from build123d import *

# Parameters (mm, degrees)
F0_W     = 100
F0_H     = 60
F1_DEPTH = 50
F2_W     = 15
F2_H     = 32
F3_DEPTH = 100.001
F4_W     = 70
F4_H     = 15
F5_DEPTH = 60.001
F6_SIZE2 = 15
F6_SIZE  = 20
F7_SIZE2 = 40
F7_SIZE  = 44


with BuildPart() as f1:
    # F0 (on Front) → F1 (new body)
    with BuildSketch(Plane.XZ):
        with Locations((50, 30)):
            Rectangle(F0_W, F0_H)
    extrude(amount=F1_DEPTH)

    # F2 (on face) → F3 (cut, through all)
    with BuildSketch(Plane.YZ.offset(100)):
        with Locations((-42.5, 16)):
            Rectangle(F2_W, F2_H)
    extrude(amount=-F3_DEPTH, mode=Mode.SUBTRACT)

    # F4 (on face) → F5 (cut, through all)
    with BuildSketch(Plane.XY.offset(60)):
        with Locations((65, -7.5)):
            Rectangle(F4_W, F4_H)
    extrude(amount=-F5_DEPTH, mode=Mode.SUBTRACT)

    # F6
    f6_edges = [f1.edges().sort_by_distance(p)[0] for p in [
        (0, -25, 60),
    ]]
    chamfer(f6_edges, length=F6_SIZE, length2=F6_SIZE2)

    # F7
    f7_edges = [f1.edges().sort_by_distance(p)[0] for p in [
        (100, -32.5, 60),
    ]]
    chamfer(f7_edges, length=F7_SIZE, length2=F7_SIZE2)


solid = f1.part
Input: part model. Units: mm. Frame: model coordinates. A direction names the side the tool comes from. Give positions to 0.01 mm unless a question says otherwise; leave off trailing zeros. Write each loop counter-clockwise with the first axis right and the second up, starting at its lowest first coordinate (ties: lowest second). Pieces come first, ordered by that corner, then holes. Notation, with made-up numbers: M 18.5,65.5 L 48.5,65.5 A15 ccw 48.5,80.5 Z; hole C 9,63.25 d4. An arc over 180 degrees is marked long. Write item = value, one per line. Start each with the question number.
1) Cut plane C-C on x = 19. Return the cut outline in (y, z), then the cut area to 3 significant figures.
2) Cut plane D-D on y = -3. Return the cut outline in (x, z), then the cut area to 3 significant figures.
3) Reachability of faces 1 (the flat face through (73.419, -32.255, 44.164)), 2 (the flat face through (51, -35, 16)), 3 (the flat face through (30, -8, 30)) from +Z, -Z, +X, -X, +Y, -Y: full face, straight path, thin tool, end or side. Return the list, or none.
4) Cut plane A-A on y = -37.5. Return the cut outline in (x, z), then the cut area to 3 significant figures.
5) Material intervals for line 1 along Z through (x, y) = (16, -45.5); line 2 along Y through (x, z) = (79.5, 35); line 3 along Y through (x, z) = (61.5, 10), sorted ascending. Write a range as [from, to].
6) Cut plane B-B on z = 25. Return the cut outline in (x, y).
7) First-contact query: pin 1 Ø3 at (y, z) = (-28, 32) entering from +X; pin 2 Ø12 at (x, y) = (35.5, -44.5) entering from -Z; pin 3 Ø1 at (y, z) = (-7.5, 44.5) entering from +X. Flat tips, straight axial feed; report the tip coordinate or a pass-through.
Solved:
q1.outline = M -50,32 L -35,32 L -35,0 L 0,0 L 0,60 L -50,60 Z
q1.area = 2,520 mm2
q2.outline = M 0,0 L 30,0 L 30,60 L 15,60 L 0,40 Z
q2.area = 1,650 mm2
q3.face_1 = +Z, +X, +Y, -Y
q3.face_2 = -Z, +X, -X, -Y
q3.face_3 = +Z, -Z, +X, +Y
q4.outline = M 0,32 L 86.8,32 L 56,60 L 15,60 L 0,40 Z
q4.area = 1,850 mm2
q5.line_1 = [32, 60]
q5.line_2 = [-50, -15]
q5.line_3 = [-35, -15]
q6.outline = M 0,-35 L 94.5,-35 L 94.5,-15 L 30,-15 L 30,0 L 0,0 Z
q7.pin_1 = 88.45
q7.pin_2 = 32
q7.pin_3 = 30
